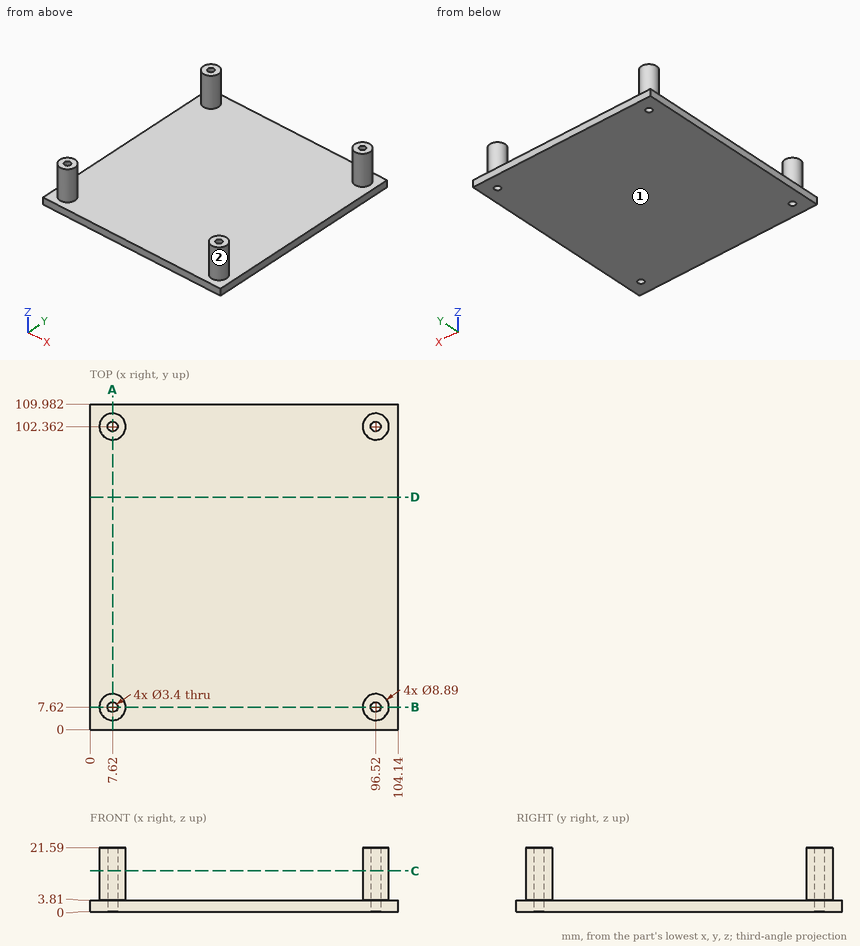
Source: three-view drawing plus pictorial views. Frame: mm from the lowest corner of the part. Round coordinates to 2 decimals unless told otherwise and drop trailing zeros. Loops run counter-clockwise (first coordinate to the right, second up) from the corner with the lowest first, then second, coordinate; pieces in that order, holes last. Notation, with made-up numbers: M -25,-29.5 L 11,-29.5 A20 cw 11,-22.5 Z; hole C 82,27 d6. An arc over 180 degrees is marked long. Put each result on its own line as item: value.
(1) Section B-B, the plane y = 7.62. Return loops of the section in (x, z) (3 decimals), and give its area (3 significant figures).
Solutions:
outline: M 0,0 L 5.92,0 L 5.92,21.59 L 3.175,21.59 L 3.175,3.81 L 0,3.81 Z; M 9.32,0 L 94.82,0 L 94.82,21.59 L 92.075,21.59 L 92.075,3.81 L 12.065,3.81 L 12.065,21.59 L 9.32,21.59 Z; M 98.22,0 L 104.14,0 L 104.14,3.81 L 100.965,3.81 L 100.965,21.59 L 98.22,21.59 Z
area: 566 mm²
(2) First-contact query: pin 1 (10 mm diameter, centred on x = 24.5, y = 93, fed in from -Z); pin 2 (1 mm diameter, centred on x = 18.5, y = 69.5, fed in from +Z). Flat tips, straight axial feed; report the tip coordinate or a pass-through.
Solutions:
pin 1: z = 0
pin 2: z = 3.81
(3) Pull-direction query (Y, two-part tool) for the marked faces 1 and 2; classes: released by +Y, released by -Y, zero draft, split by the parting line, or undercut.
Solutions:
face 1: zero draft
face 2: undercut
(4) Section C-C, the plane z = 13.75. Return loops of the section in (x, y) (3 decimals), and give its area (3 significant figures).
Solutions:
outline: C 7.62,7.62 d8.89; C 7.62,102.362 d8.89; C 96.52,7.62 d8.89; C 96.52,102.362 d8.89; hole C 7.62,7.62 d3.4; hole C 7.62,102.362 d3.4; hole C 96.52,7.62 d3.4; hole C 96.52,102.362 d3.4
area: 212 mm²
(5) Section A-A, the plane x = 7.62. Return loops of the section in (y, z) (3 decimals).
Solutions:
outline: M 0,0 L 5.92,0 L 5.92,21.59 L 3.175,21.59 L 3.175,3.81 L 0,3.81 Z; M 9.32,0 L 100.662,0 L 100.662,21.59 L 97.917,21.59 L 97.917,3.81 L 12.065,3.81 L 12.065,21.59 L 9.32,21.59 Z; M 104.062,0 L 109.982,0 L 109.982,3.81 L 106.807,3.81 L 106.807,21.59 L 104.062,21.59 Z
(6) Ray query, line 1 (Y direction, x = 96.52, z = 10.75) (3 decimals); line 2 (X direction, y = 101, z = 17.5); line 3 (Z direction, x = 45, y = 15). Return the intervals inside material, ascending. Write a range as [from, to].
Solutions:
line 1: [3.175, 5.92], [9.32, 12.065], [97.917, 100.662], [104.062, 106.807]
line 2: [3.39, 6.6], [8.64, 11.85], [92.29, 95.5], [97.54, 100.75]
line 3: [0, 3.81]
(7) Section D-D, the plane y = 78.5. Return loops of the section in (x, z), and give its area (3 significant figures).
Solutions:
outline: M 0,0 L 104.14,0 L 104.14,3.81 L 0,3.81 Z
area: 397 mm²
